Autodesk Inventor part; units mm, degrees
ref_plane "YZ Plane" through (0, 0, 0) normal (1, 0, 0) x (0, 1, 0)
ref_plane "XZ Plane" through (0, 0, 0) normal (0, 1, 0) x (-1, 0, 0)
ref_plane "XY Plane" through (0, 0, 0) normal (0, 0, 1) x (1, 0, 0)
sketch "Sketch1" plane through (0, 0, 0) normal (0, 1, 0) x (-1, 0, 0)
  line L0 (0, 0.9) -> (0, -0.9)
  line L1 (0, -0.9) -> (-2.75, -0.9)
  line L2 (-3.1754, -0.6544) -> (-3.1754, 0.6544)
  line L3 (-2.75, 0.9) -> (0, 0.9)
  line L4 (-2.75, 0.9) -> (-3.1754, 0.6544)
  line L5 (-2.75, -0.9) -> (-3.1754, -0.6544)
  line L6 (0, 0) -> (-3.1754, 0) construction
  dimension "d0" = 1.8
  dimension "d1" = 5.5
  dimension "d2" = 6.3509
  dimension "d3" = 30
revolve "Revolution1" add sketch "Sketch1" angle 360 about axis through (0, 0, 0.9) along (0, 0, -1)
sketch "Sketch2" plane through (0, 0, 0.9) normal (0, 0, 1) x (1, 0, 0)
  circle A0 centre (0, 0) radius 3.1754
  line L0 (0, 3.1754) -> (2.75, 1.5877)
  line L1 (2.75, 1.5877) -> (2.75, -1.5877)
  line L2 (2.75, -1.5877) -> (0, -3.1754)
  line L3 (0, -3.1754) -> (-2.75, -1.5877)
  line L4 (-2.75, -1.5877) -> (-2.75, 1.5877)
  line L5 (-2.75, 1.5877) -> (0, 3.1754)
  point P0 (0, 0)
  point P1 (0, 0)
  point P2 (0, 0)
  point P3 (-2.75, -1.5877)
  point P4 (-2.75, -1.5877)
  point P5 (0, -3.1754)
  point P6 (0, -3.1754)
extrude "Extrusion1" cut sketch "Sketch2" against normal through all contours A0 L1 | L0 A0 | A0 L2 | L5 A0 | A0 L3 | L4 A0
hole "Hole1" at (0, 0, 0.9) direction (0, 0, -1) diameter 2.459 depth 6 countersink diameter 3 countersink angle 90
mirror "Mirror1" about plane through (0, 0, 0) normal (0, 0, 1) of "Hole1"
equation "\"d2\" = 1.1547 * d1"
properties part number "UNT-03-3" material "Stainless Steel AISI 304"
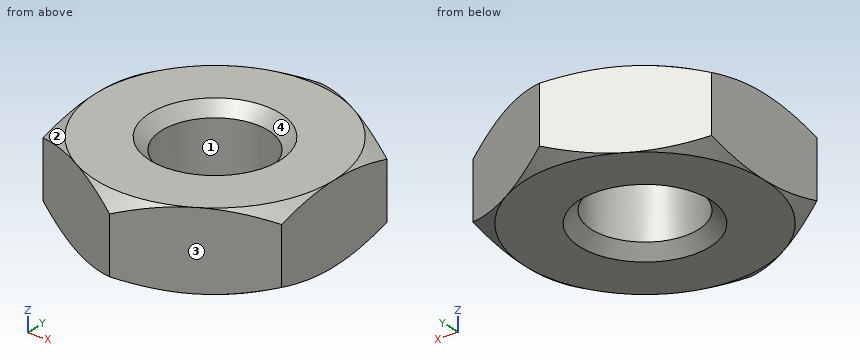
For this review, take the finished solid that the model builds, in its own axes (mm). Face numbers are marked on the shaded views. Coordinates: 2 decimals unless noted, no trailing zeros. Loops run counter-clockwise (first coordinate to the right, second up) from the corner with the lowest first, then second, coordinate; pieces in that order, holes last.
1. For line 1 (X direction, y = 0, z = 0.3); line 2 (Y direction, x = -0.1, z = 0.75); line 3 (X direction, y = -0.5, z = -0.3), list the stretches that pass through material, from the lowest coordinate up.
2. Add section A-A, the plane z = 0.55. Give the boundary of the cut face in (x, y).
3. Insertion check: P1, Ø1.5, axis at x = 2, y = -2, coming from the +Z side; P2, Ø1.5, axis at x = 0, y = 0, coming from the +Z side. Each pin has a flat end and moves straight along its axis. Give the tip position at first contact, or say it passes through.
4. Mouldability with a two-part tool opening along X and no side actions: class the marked faces 1, 2, 3 and 4 as +X half, -X half, draft (parallel to the pull), parting line (faces both ways), or undercut.
Result:
1. line 1: x = -2.75 to -1.23, 1.23 to 2.75
1. line 2: y = -3.01 to -1.35, 1.35 to 3.01
1. line 3: x = -2.75 to -1.12, 1.12 to 2.75
2. outline: (-2.75, -1.59) - (0, -3.18) - (2.75, -1.59) - (2.75, 1.59) - (0, 3.18) - (-2.75, 1.59) - close; hole circle Ø2.46 at (0, 0)
3. P1: stops at z = 0.9
3. P2: passes through
4. face 1: undercut
4. face 2: -X half
4. face 3: +X half
4. face 4: undercut
